Part model, mm, in its own coordinate system. A direction names the side the tool comes from. Give positions to 0.01 mm unless a question says otherwise; leave off trailing zeros. Order: outer loops, then holes, each group sorted by start corner. A loop starts at its lowest first (then second) coordinate and runs counter-clockwise, first axis right, second up. Notation, with made-up numbers: M -30.5,79.25 L -24.5,79.25 A22 ccw -24.5,93.25 Z; hole C 25.5,31 d3. An arc over 180 degrees is marked long. One line per question, with ' | ' between items.
```python
from build123d import *

# Parameters (mm, degrees)
SKETCH1_W                   = 369
SKETCH1_H                   = 200
BOSS_EXTRUDE1_DEPTH         = 20
SKETCH2_W                   = 129
SKETCH2_H                   = 16
BOSS_EXTRUDE2_DEPTH         = 10
SKETCH3_W                   = 342
SKETCH3_H                   = 168
CUT_EXTRUDE1_DEPTH          = 9
SKETCH4_W                   = 100
SKETCH4_H                   = 10
BOSS_EXTRUDE3_DEPTH         = 60
CUT_EXTRUDE3_DEPTH          = 10
CUT_EXTRUDE3_DEPTH_BACK     = 60
SKETCH10_W                  = 404
SKETCH10_H                  = 324.796202869
CUT_EXTRUDE4_DEPTH          = 69
CUT_EXTRUDE7_DEPTH          = 274.752168941
CUT_EXTRUDE7_DEPTH_BACK     = 274.752168941
SKETCH14_W                  = 37
SKETCH14_H                  = 34.717467541
SKETCH12_W                  = 50
SKETCH12_H                  = 11
BOSS_EXTRUDE6_DEPTH         = 20
SKETCH13_R                  = 4
CUT_EXTRUDE6_DEPTH          = 229.43215623
CORTAR_EXTRUIR4_DEPTH       = 220
CROQUIS5_W                  = 20
CROQUIS5_H                  = 11
SALIENTE_EXTRUIR2_DEPTH     = 10
CROQUIS6_W                  = 20
CROQUIS6_H                  = 11
SALIENTE_EXTRUIR3_DEPTH     = 20
CROQUIS8_R                  = 5
CORTAR_EXTRUIR5_DEPTH       = 48
CROQUIS9_W                  = 38
CROQUIS9_H                  = 65
CORTAR_EXTRUIR6_DEPTH       = 85
CROQUIS10_W                 = 10
CROQUIS10_H                 = 16
SALIENTE_EXTRUIR4_DEPTH     = 7.89
CROQUIS11_W                 = 16
CROQUIS11_H                 = 19
SALIENTE_EXTRUIR5_DEPTH     = 13
CORTAR_EXTRUIR10_DEPTH      = 36.9
CORTAR_EXTRUIR10_DEPTH_BACK = 7.894953
CROQUIS12_W                 = 18
CROQUIS12_H                 = 16
CROQUIS13_W                 = 5
CROQUIS13_H                 = 16
CORTAR_EXTRUIR11_DEPTH      = 19
CROQUIS14_W                 = 25
CROQUIS14_H                 = 11
SALIENTE_EXTRUIR6_DEPTH     = 20
CROQUIS15_W                 = 20
CROQUIS15_H                 = 25
CORTAR_EXTRUIR12_DEPTH      = 238.868135739
CROQUIS16_R                 = 5
CORTAR_EXTRUIR13_DEPTH      = 238.868135739
CROQUIS17_W                 = 20
CROQUIS17_H                 = 20
SALIENTE_EXTRUIR7_DEPTH     = 11
CROQUIS18_W                 = 20
CROQUIS18_H                 = 20
CORTAR_EXTRUIR14_DEPTH      = 238.868135739
CROQUIS19_R                 = 5
CORTAR_EXTRUIR15_DEPTH      = 229.43215623


with BuildPart() as part:
    # Sketch1 → Boss-Extrude1 (new body)
    with BuildSketch(Plane(origin=(0, 0, 0), x_dir=(1, 0, 0), z_dir=(0, 1, 0))):
        Rectangle(SKETCH1_W, SKETCH1_H)
    extrude(amount=BOSS_EXTRUDE1_DEPTH)

    # Sketch2 → Boss-Extrude2 (add)
    with BuildSketch(Plane(origin=(0, 20, 0), x_dir=(1, 0, 0), z_dir=(0, 1, 0))):
        Polygon((-184.5, -100), (-169.5, -100), (-119.5, -100), (-119.5, -84), (-169.5, -84), (-169.5, -35), (-184.5, -35), align=None)
        Polygon((-184.5, 100), (-169.5, 100), (-119.5, 100), (-119.5, 84), (-169.5, 84), (-169.5, 35), (-184.5, 35), align=None)
        with Locations((20, -92)):
            Rectangle(SKETCH2_W, SKETCH2_H)
        with Locations((20, 92)):
            Rectangle(SKETCH2_W, SKETCH2_H)
    extrude(amount=BOSS_EXTRUDE2_DEPTH)

    # Sketch3 → Cut-Extrude1 (cut)
    with BuildSketch(Plane(origin=(0, 20, 0), x_dir=(1, 0, 0), z_dir=(0, 1, 0))):
        with Locations((1.5, 0)):
            Rectangle(SKETCH3_W, SKETCH3_H)
    extrude(amount=-CUT_EXTRUDE1_DEPTH, mode=Mode.SUBTRACT)

    # Sketch4 → Boss-Extrude3 (add)
    with BuildSketch(Plane(origin=(0, 0, -100), x_dir=(-1, 0, 0), z_dir=(0, 0, -1))):
        with Locations((-19.5, 25)):
            Rectangle(SKETCH4_W, SKETCH4_H)
    extrude(amount=BOSS_EXTRUDE3_DEPTH)

    # Sketch6 → Cut-Extrude3 (cut, two sides: drawn at the far end of the back side and taken through both)
    with BuildSketch(Plane.XY.offset(-84).offset(-CUT_EXTRUDE3_DEPTH_BACK)):
        with BuildLine():
            Line((-24.5, 30), (-26.030765637, 28.081051534))
            ThreePointArc((-26.030765637, 28.081051534), (-26.158442873, 26.948989892), (-25.193843525, 26.342843758))
            Line((-25.193843525, 26.342843758), (-15.806155854, 26.342843758))
            ThreePointArc((-15.806155854, 26.342843758), (-14.841556992, 26.948990172), (-14.969234363, 28.081051534))
            Line((-14.969234363, 28.081051534), (-16.5, 30))
            Line((-16.5, 30), (-24.5, 30))
        make_face()
        with BuildLine():
            Line((56.5, 30), (54.981983491, 27.801494438))
            ThreePointArc((54.981983491, 27.801494438), (54.9192914, 26.767046688), (55.80615587, 26.230871478))
            Line((55.80615587, 26.230871478), (65.193843541, 26.230871478))
            ThreePointArc((65.193843541, 26.230871478), (66.080708464, 26.767046428), (66.018016509, 27.801494438))
            Line((66.018016509, 27.801494438), (64.5, 30))
            Line((64.5, 30), (56.5, 30))
        make_face()
    extrude(amount=CUT_EXTRUDE3_DEPTH + CUT_EXTRUDE3_DEPTH_BACK, mode=Mode.SUBTRACT)

    # Sketch10 → Cut-Extrude4 (cut)
    with BuildSketch(Plane(origin=(0, 30, 0), x_dir=(1, 0, 0), z_dir=(0, 1, 0))):
        with Locations((55.5, -0.89352463)):
            Rectangle(SKETCH10_W, SKETCH10_H)
    extrude(amount=-CUT_EXTRUDE4_DEPTH, mode=Mode.SUBTRACT)

    # Sketch14 → Cut-Extrude7 (cut, two sides: drawn at the far end of the back side and taken through both)
    with BuildSketch(Plane(origin=(0, 0, -100), x_dir=(-1, 0, 0), z_dir=(0, 0, -1)).offset(-CUT_EXTRUDE7_DEPTH_BACK)):
        with Locations((138, 36.253686327)):
            Rectangle(SKETCH14_W, SKETCH14_H)
    extrude(amount=CUT_EXTRUDE7_DEPTH + CUT_EXTRUDE7_DEPTH_BACK, mode=Mode.SUBTRACT)

    # Sketch12 → Boss-Extrude6 (add)
    with BuildSketch(Plane.ZY.offset(184.5)):
        with Locations((-25, 5.5)):
            Rectangle(SKETCH12_W, SKETCH12_H)
    extrude(amount=BOSS_EXTRUDE6_DEPTH)

    # Sketch13 → Cut-Extrude6 (cut, through all)
    with BuildSketch(Plane(origin=(0, 11, 0), x_dir=(1, 0, 0), z_dir=(0, 1, 0))):
        with Locations(Location((-194.5, 25, 0), (0, 0, 270))):
            Circle(SKETCH13_R)
    extrude(amount=-CUT_EXTRUDE6_DEPTH, mode=Mode.SUBTRACT)

    # Croquis3 → Cortar-Extruir4 (cut)
    with BuildSketch(Plane(origin=(0, 30, 0), x_dir=(1, 0, 0), z_dir=(0, 1, 0))):
        Polygon((-169.5, -35), (-146.5, -35), (-146.5, 0), (-146.5, 35), (-204.5, 35), (-204.5, 0), (-204.5, -35), (-184.5, -35), align=None)
    extrude(amount=-CORTAR_EXTRUIR4_DEPTH, mode=Mode.SUBTRACT)


with BuildPart() as cortar_extruir4_piece_1:
    # of the separate pieces the step leaves, piece 1, a body of its own (cortar_extruir4_pieces)
    add(part.part.solids().sort_by_distance((-184.5, 30, -100))[0])

    # Croquis5 → Saliente-Extruir2 (add)
    with BuildSketch(Plane(origin=(0, 0, -50), x_dir=(-1, 0, 0), z_dir=(0, 0, -1))):
        with Locations((194.5, 5.5)):
            Rectangle(CROQUIS5_W, CROQUIS5_H)
    extrude(amount=SALIENTE_EXTRUIR2_DEPTH)

    # Croquis6 → Saliente-Extruir3 (add)
    with BuildSketch(Plane(origin=(0, 0, -100), x_dir=(-1, 0, 0), z_dir=(0, 0, -1))):
        with Locations((174.5, 5.5)):
            Rectangle(CROQUIS6_W, CROQUIS6_H)
    extrude(amount=SALIENTE_EXTRUIR3_DEPTH)

    # Croquis8 → Cortar-Extruir5 (cut)
    with BuildSketch(Plane(origin=(0, 11, 0), x_dir=(1, 0, 0), z_dir=(0, 1, 0))):
        with Locations(Location((-194.5, 47.5, 0), (0, 0, 270))):
            Circle(CROQUIS8_R)
        with Locations((-194.5, -47.5)):
            Circle(CROQUIS8_R)
        with Locations((-174.5, -110)):
            Circle(CROQUIS8_R)
        with Locations(Location((-174.5, 110, 0), (0, 0, 270))):
            Circle(CROQUIS8_R)
    extrude(amount=-CORTAR_EXTRUIR5_DEPTH, mode=Mode.SUBTRACT)

    # Croquis10 → Saliente-Extruir4 (add)
    with BuildSketch(Plane(origin=(0, 11, 0), x_dir=(1, 0, 0), z_dir=(0, 1, 0))):
        with Locations((-151.5, 43)):
            Rectangle(CROQUIS10_W, CROQUIS10_H)
    extrude(amount=SALIENTE_EXTRUIR4_DEPTH)

    # Croquis11 → Saliente-Extruir5 (add)
    with BuildSketch(Plane(origin=(-169.5, 0, 0), x_dir=(0, 0, -1), z_dir=(1, 0, 0))):
        with Locations((43, 20.5)):
            Rectangle(CROQUIS11_W, CROQUIS11_H)
    extrude(amount=SALIENTE_EXTRUIR5_DEPTH)

    # Croquis12 → Cortar-Extruir10 (cut, two sides: drawn at the far end of the back side and taken through both)
    with BuildSketch(Plane(origin=(0, 18.894952557, 0), x_dir=(1, 0, 0), z_dir=(0, 1, 0)).offset(-CORTAR_EXTRUIR10_DEPTH_BACK)):
        with Locations((-155.5, 92)):
            Rectangle(CROQUIS12_W, CROQUIS12_H)
    extrude(amount=CORTAR_EXTRUIR10_DEPTH + CORTAR_EXTRUIR10_DEPTH_BACK, mode=Mode.SUBTRACT)

    # Croquis13 → Cortar-Extruir11 (cut)
    with BuildSketch(Plane(origin=(0, 30, 0), x_dir=(1, 0, 0), z_dir=(0, 1, 0))):
        with Locations((-167, 92)):
            Rectangle(CROQUIS13_W, CROQUIS13_H)
    extrude(amount=-CORTAR_EXTRUIR11_DEPTH, mode=Mode.SUBTRACT)

    # Croquis14 → Saliente-Extruir6 (add)
    with BuildSketch(Plane.ZY.offset(184.5)):
        with Locations((-87.5, 5.5)):
            Rectangle(CROQUIS14_W, CROQUIS14_H)
    extrude(amount=SALIENTE_EXTRUIR6_DEPTH)

    # Croquis15 → Cortar-Extruir12 (cut, through all)
    with BuildSketch(Plane(origin=(0, 11, 0), x_dir=(1, 0, 0), z_dir=(0, 1, 0))):
        with Locations((-194.5, 47.5)):
            Rectangle(CROQUIS15_W, CROQUIS15_H)
    extrude(amount=-CORTAR_EXTRUIR12_DEPTH, mode=Mode.SUBTRACT)

    # Croquis16 → Cortar-Extruir13 (cut, through all)
    with BuildSketch(Plane(origin=(0, 11, 0), x_dir=(1, 0, 0), z_dir=(0, 1, 0))):
        with Locations(Location((-194.5, 87.5, 0), (0, 0, 270))):
            Circle(CROQUIS16_R)
    extrude(amount=-CORTAR_EXTRUIR13_DEPTH, mode=Mode.SUBTRACT)

    # Croquis17 → Saliente-Extruir7 (add)
    with BuildSketch(Plane(origin=(0, 11, 0), x_dir=(1, 0, 0), z_dir=(0, 1, 0))):
        with Locations((-174.5, 25)):
            Rectangle(CROQUIS17_W, CROQUIS17_H)
    extrude(amount=-SALIENTE_EXTRUIR7_DEPTH)

    # Croquis18 → Cortar-Extruir14 (cut, through all)
    with BuildSketch(Plane(origin=(0, 11, 0), x_dir=(1, 0, 0), z_dir=(0, 1, 0))):
        with Locations((-174.5, 110)):
            Rectangle(CROQUIS18_W, CROQUIS18_H)
    extrude(amount=-CORTAR_EXTRUIR14_DEPTH, mode=Mode.SUBTRACT)

    # Croquis19 → Cortar-Extruir15 (cut, through all)
    with BuildSketch(Plane(origin=(0, 11, 0), x_dir=(1, 0, 0), z_dir=(0, 1, 0))):
        with Locations(Location((-174.5, 25, 0), (0, 0, 270))):
            Circle(CROQUIS19_R)
    extrude(amount=-CORTAR_EXTRUIR15_DEPTH, mode=Mode.SUBTRACT)


with BuildPart() as cortar_extruir4_piece_2:
    # of the separate pieces the step leaves, piece 2, a body of its own (cortar_extruir4_pieces)
    add(part.part.solids().sort_by_distance((-184.5, 30, 100))[0])

    # Croquis9 → Cortar-Extruir6 (cut)
    with BuildSketch(Plane(origin=(0, 30, 0), x_dir=(1, 0, 0), z_dir=(0, 1, 0))):
        with Locations((-165.5, -67.5)):
            Rectangle(CROQUIS9_W, CROQUIS9_H)
    extrude(amount=-CORTAR_EXTRUIR6_DEPTH, mode=Mode.SUBTRACT)


solid = cortar_extruir4_piece_1.part
```
1. Probe L1, parallel to X at y = 6, z = -25; L2, parallel to X at y = 5, z = -87.5; L3, parallel to Y at x = -160, z = -80.5. List the from-to ranges inside material, lowest first. Write a range as from..to.
Worked out:
L1: x = -184.5..-179.5, -169.5..-164.5 | L2: x = -204.5..-199.5, -189.5..-146.5 | L3: y = 0..11
2. Slice it at A-A on z = -87.5. Give the cut face in (x, y), then the cut area to 3 significant figures.
Worked out:
outline: M -204.5,0 L -199.5,0 L -199.5,11 L -204.5,11 Z; M -189.5,0 L -146.5,0 L -146.5,11 L -169.5,11 L -169.5,30 L -184.5,30 L -184.5,11 L -189.5,11 Z | area: 813 mm2
3. Slice it at D-D on x = -158. Give the cut face in (y, z).
Worked out:
outline: M 0,-100 L 11,-100 L 11,-51 L 30,-51 L 30,-35 L 0,-35 Z
4. Tool access for faces 1 (the flat face through (-194, 5, -75)), 2 (the flat face through (-189.9, 11, -84.9)), 3 (the flat face through (-164.5, 6, -25)): list every direction of +Z, -Z, +X, -X, +Y, -Y with a clear straight run to the whole face (end or side of a thin tool).
Worked out:
face 1: +Z, -X, +Y, -Y | face 2: +Z, -Z, -X, +Y | face 3: +Z, +X, +Y, -Y
5. Drop flat-ended pins along their axis: pin 1 (3 mm diameter, centred on x = -187, z = -82, fed in from +Y); pin 2 (1.5 mm diameter, centred on x = -196.5, y = 9, fed in from +Z); pin 3 (5 mm diameter, centred on x = -166.5, y = 17, fed in from +Z); pin 4 (6 mm diameter, centred on x = -197, y = 16.5, fed in from +Z). Give the stop position or say it passes through.
Worked out:
pin 1: stops at y = 11 | pin 2: stops at z = -75 | pin 3: stops at z = -35 | pin 4: passes through
6. Mould opens along X. For faces 4 (the flat face through (-176, 8, -100)), 5 (the flat face through (-146.5, 7, -60)), 6 (the cylindrical face through (-169.543, 5.577, -25.651)) say: released by +X, released by -X, zero draft, split by the parting line, or undercut.
Worked out:
face 4: zero draft | face 5: released by +X | face 6: undercut
7. Slice it at C-C on y = 4.75. Give the cut face in (x, z).
Worked out:
outline: M -204.5,-100 L -146.5,-100 L -146.5,-35 L -164.5,-35 L -164.5,-15 L -184.5,-15 L -184.5,-75 L -204.5,-75 Z; hole C -194.5,-87.5 d10; hole C -174.5,-25 d10
8. Slice it at B-B on x = -194.5. Give the cut face in (y, z).
Worked out:
outline: M 0,-100 L 11,-100 L 11,-92.5 L 0,-92.5 Z; M 0,-82.5 L 11,-82.5 L 11,-75 L 0,-75 Z
